from build123d import *

# Parameters (mm, degrees)
SKETCH2_R           = 1.190625
BOSS_EXTRUDE1_DEPTH = 1.5875
FILLET1_SIZE        = 3.175


with BuildPart() as part:
    # Sketch2 → Boss-Extrude1 (new body)
    with BuildSketch(Plane(origin=(0, 0, 0), x_dir=(1, 0, 0), z_dir=(0, 1, 0))):
        Polygon((29.393690453, -107.736776908), (34.156190453, -101.788416314), (34.156190453, 31.968309197), (28.155939525, 36.772354713), (23.075939525, 36.772354713), (20.099377025, 33.054629342), (29.393690453, 25.613223092), (20.099377025, 14.004629342), (24.746533739, 10.283926217), (29.393690453, 6.563223092), (20.099377025, -5.045370658), (29.393690453, -12.486776908), (20.099377025, -24.095370658), (29.393690453, -31.536776908), (20.099377025, -43.145370658), (29.393690453, -50.586776908), (20.099377025, -62.195370658), (29.393690453, -69.636776908), (20.099377025, -81.245370658), (29.393690453, -88.686776908), (20.099377025, -100.295370658), align=None)
        with Locations(Location((26.234814989, -102.157211097, 0), (0, 0, 270))):
            Circle(SKETCH2_R, mode=Mode.SUBTRACT)
        with Locations(Location((26.234814989, -83.107211097, 0), (0, 0, 270))):
            Circle(SKETCH2_R, mode=Mode.SUBTRACT)
        with Locations(Location((26.234814989, -64.057211097, 0), (0, 0, 270))):
            Circle(SKETCH2_R, mode=Mode.SUBTRACT)
        with Locations(Location((26.234814989, -45.007211097, 0), (0, 0, 270))):
            Circle(SKETCH2_R, mode=Mode.SUBTRACT)
        with Locations(Location((26.234814989, -25.957211097, 0), (0, 0, 270))):
            Circle(SKETCH2_R, mode=Mode.SUBTRACT)
        with Locations(Location((26.234814989, -6.907211097, 0), (0, 0, 270))):
            Circle(SKETCH2_R, mode=Mode.SUBTRACT)
        with BuildLine():
            ThreePointArc((27.425439989, 12.142788903), (26.750370737, 11.069574031), (25.490674364, 11.21335756))
            ThreePointArc((25.490674364, 11.21335756), (25.719259241, 13.216003775), (27.425439989, 12.142788903))
        make_face(mode=Mode.SUBTRACT)
        with Locations(Location((26.234814989, 31.192788903, 0), (0, 0, 270))):
            Circle(SKETCH2_R, mode=Mode.SUBTRACT)
    extrude(amount=BOSS_EXTRUDE1_DEPTH)

    # Fillet1
    # a fillet whose section is not a circle: 3.175 mm, written as the material it takes off along each edge
    with BuildSketch(Plane(origin=(29.393690453, -7.9375, 107.736776908), x_dir=(0.6249999999921612, 0, -0.7806247498060759), z_dir=(0, 1, 0))) as fillet1_piece_1:
        with BuildLine():
            Bezier((FILLET1_SIZE, 0), (0, 0), (0, FILLET1_SIZE), weights=[1, 0.224506403, 1])
            Line((0, FILLET1_SIZE), (0, 0))
            Line((0, 0), (FILLET1_SIZE, 0))
        make_face()
    extrude(amount=17.4625, mode=Mode.SUBTRACT)
    with BuildSketch(Plane(origin=(34.156190453, -2.786065678, 101.788416314), x_dir=(-0.6250000000189532, 0, 0.7806247497846253), z_dir=(0, 1, 0))) as fillet1_piece_2:
        with BuildLine():
            Bezier((1.114426271, 0), (0, 0), (-0.869948729, -0.696516419), weights=[1, 0.299581461, 1])
            Line((-0.869948729, -0.696516419), (0, 0))
            Line((0, 0), (1.114426271, 0))
        make_face()
    extrude(amount=7.159631356, mode=Mode.SUBTRACT)
    with BuildSketch(Plane(origin=(34.156190453, -3.813051663, -31.968309197), x_dir=(-0.7806247498123451, 0, -0.624999999984331), z_dir=(0, 1, 0)), Plane(origin=(23.075939525, -3.813051662, -36.772354713), x_dir=(-0.6250000000000002, 0, 0.7806247497997996), z_dir=(0, 1, 0))) as fillet1_piece_3:
        with BuildLine():
            Bezier((1.525220665, 0), (0, 0), (-0.953262916, 1.190625), weights=[1, 0.286190632, 1])
            Line((-0.953262916, 1.190625), (0, 0))
            Line((0, 0), (1.525220665, 0))
        make_face()
    extrude(amount=9.213603325, mode=Mode.SUBTRACT)
    with BuildSketch(Plane(origin=(28.155939525, -2.786065678, -36.772354713), x_dir=(-1, 0, 0), z_dir=(0, 1, 0))) as fillet1_piece_4:
        with BuildLine():
            Bezier((1.114426271, 0), (0, 0), (-0.869948729, 0.696516419), weights=[1, 0.299581461, 1])
            Line((-0.869948729, 0.696516419), (0, 0))
            Line((0, 0), (1.114426271, 0))
        make_face()
    extrude(amount=7.159631355, mode=Mode.SUBTRACT)


solid = part.part
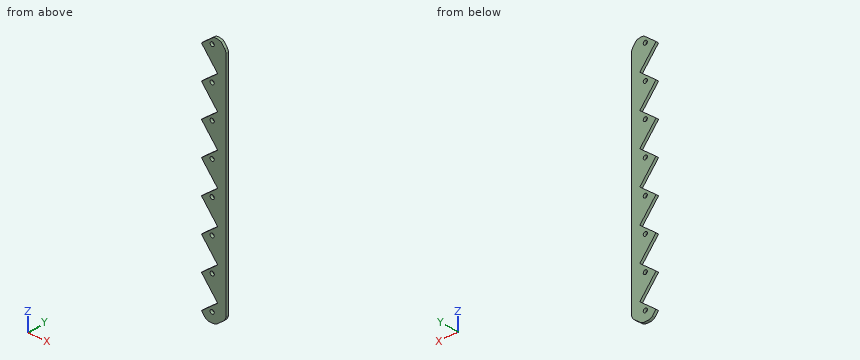
Verification items for the finished model (mm, model axes). Coordinates: 2 decimals unless noted, no trailing zeros. Loops run counter-clockwise (first coordinate to the right, second up) from the corner with the lowest first, then second, coordinate; pieces in that order, holes last. Notation, with made-up numbers: (-5, 59) -> (3, 59) arc R11 cw to (3, 64) -> close; hole circle Ø2 at (77.25, -4.75). An arc over 180 degrees is marked (long way). Answer as a JSON object with one key per item and string values. Group by question number.
Item 1: Sectioned sample at B-B on z = 75. Record the boundary of the cut face in (x, y), plus the area to 3 significant figures.
Item 2: Scan lines: probe 1 along X at (y, z) = (0.3, 74.5); probe 2 along X at (y, z) = (0.7, -19); probe 3 along Z at (x, y) = (33.75, 0.7). Record each from-to range of solid material in increasing order.
Item 3: Sectioned sample at C-C on z = 30. Record the boundary of the cut face in (x, y).
Item 4: Sectioned sample at A-A on y = 0.4. State how many separate pieces and enclosed holes the cut face has, plus the area to 3 significant figures.
Evaluation:
{
 "1": {"outline": "(25.1, 0) -> (34.16, 0) -> (34.16, 1.59) -> (25.1, 1.59) -> close", "area": "14.4 mm²"},
 "2": {"probe 1": "x = 25.5 to 34.16", "probe 2": "x = 24.1 to 34.16", "probe 3": "z = -31.63 to 102.06"},
 "3": {"outline": "(27.47, 0) -> (34.16, 0) -> (34.16, 1.59) -> (27.47, 1.59) -> close"},
 "4": {"separate pieces": "1", "enclosed holes": "8", "area": "1,300 mm²"}
}
